Study the drawing (mm; zero at the part's minimum x, y, z) and answer. A direction names the side the tool comes from. Round coordinates to 2 decimals unless told otherwise and drop trailing zeros. Loops run counter-clockwise (first coordinate to the right, second up) from the corner with the lowest first, then second, coordinate; pieces in that order, holes last. Notation, with made-up numbers: (30.5, -6) - (44.5, -6) arc R23 ccw to (44.5, 11) - close; hole circle Ø1 at (57.25, -2). An arc over 180 degrees is marked (long way). Use CSV: the item, a comma, the result in double quotes. Start each with the question number.
1. A tool of negligible diameter and unlimited length cuts with its end or side. For the marked faces 5 and 6, from which of +Z, -Z, +X, -X, +Y, -Y can it reach the whole face along a straight path? Write none if from no direction.
2. Consider line 1 along Z through (x, y) = (88, 45.5); line 2 along X through (y, z) = (33, 21.5); line 3 along Y through (x, z) = (31.5, 11). Determine where each line is inside the solid, lowest interval first.
3. Find section B-B (x = 21). Give the vertices of the cut face in (y, z).
4. Find section C-C (y = 14). Give the vertices of the cut face in (x, z).
5. Given pin 1 Ø6 at (x, y) = (67.5, 6.5) entering from +Z; pin 2 Ø1 at (x, y) = (39, 42) entering from -Z; pin 3 Ø2 at (x, z) = (47.5, 39.5) entering from -Y, each flat-ended and moving along its own axis, determine where each tip first touches the part or whether it passes through.
6. Find section A-A (y = 28). Give the vertices of the cut face in (x, z).
7. Find section D-D (z = 30.5). Give the vertices of the cut face in (x, y), and give its area (3 significant figures).
8. Determine the mould class of the marked faces 1, 2, 3 and 4 for opening direction Z: +Z half, -Z half, draft (parallel to the pull), parting line (faces both ways), or undercut.
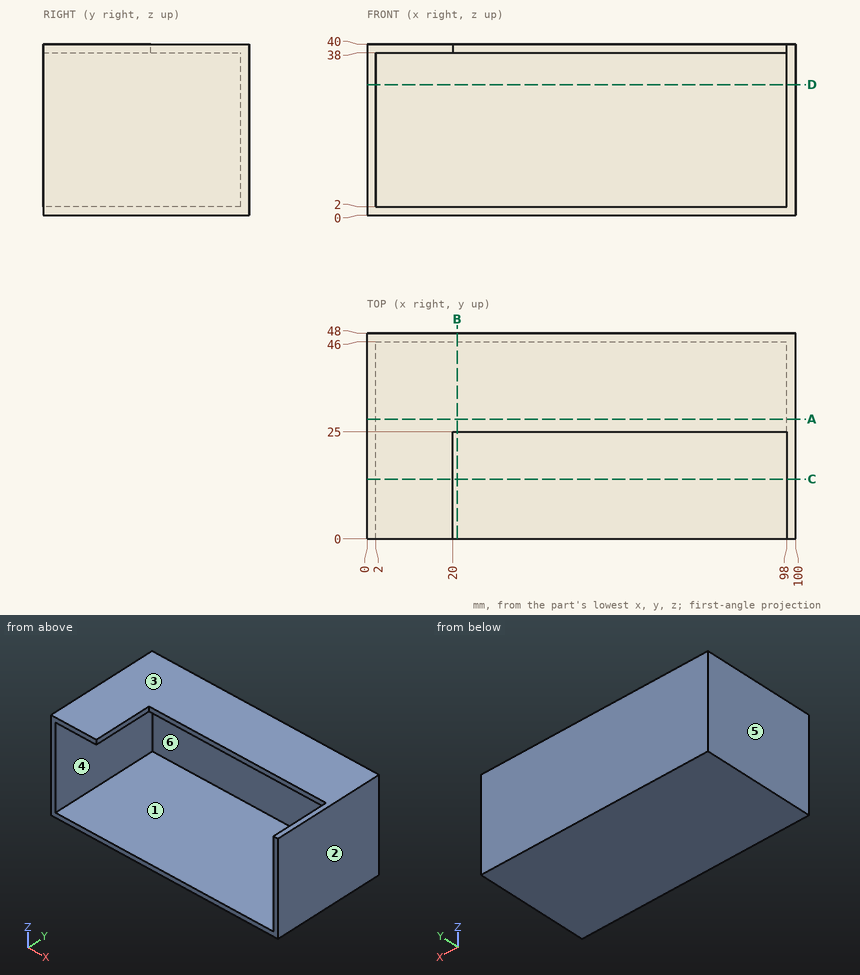
Filled sheet:
1,face 5,"+Z, -Z, -X, +Y, -Y"
1,face 6,"-Y"
2,line 1,"z = 0 to 2, 38 to 40"
2,line 2,"x = 0 to 2, 98 to 100"
2,line 3,"y = 46 to 48"
3,outline,"(0, 0) - (48, 0) - (48, 40) - (25, 40) - (25, 38) - (46, 38) - (46, 2) - (0, 2) - close"
4,outline,"(0, 0) - (100, 0) - (100, 40) - (98, 40) - (98, 2) - (2, 2) - (2, 38) - (20, 38) - (20, 40) - (0, 40) - close"
5,pin 1,"stops at z = 2"
5,pin 2,"stops at z = 0"
5,pin 3,"stops at y = 25"
6,outline,"(0, 0) - (100, 0) - (100, 40) - (0, 40) - close; hole (2, 2) - (98, 2) - (98, 38) - (2, 38) - close"
7,outline,"(0, 0) - (2, 0) - (2, 46) - (98, 46) - (98, 0) - (100, 0) - (100, 48) - (0, 48) - close"
7,area,"384 mm²"
8,face 1,"undercut"
8,face 2,"draft"
8,face 3,"+Z half"
8,face 4,"undercut"
